Work out the finished part from the listing and answer in its coordinate system (mm). A direction names the side the tool comes from. Coordinates: 2 decimals unless noted, no trailing zeros. Order: outer loops, then holes, each group sorted by start corner. A loop starts at its lowest first (then second) coordinate and runs counter-clockwise, first axis right, second up. Notation, with made-up numbers: (32.5, 59) -> (59.5, 59) arc R29 cw to (59.5, 83) -> close; hole circle Ø6 at (66, -10.5). An arc over 180 degrees is marked (long way). Answer as CSV lines item,"result". Start each with the question number.
Item 1: Section A-A (y = -1.75) is taken. Write down the section's boundary in (x, z) (3 decimals).
Item 2: For a pull along Z with two mould halves and no side action, classify faces 1 (the face through (2.244, -4.072, 8.875)), 2 (the face through (6, -3, -28.575)), 3 (the face through (-5.08, -2, -5)) as pulls with the +Z half, pulls with the -Z half, needs draft (parallel to the pull), parting line crosses it, or undercut.
Item 3: Section D-D (y = 6.5) is taken. Write down the section's boundary in (x, z) (3 decimals).
Item 4: Which of the six approach directions +Z, -Z, +X, -X, +Y, -Y give full straight-line access (tool end or side, diameter ignored) to faces 4 (the face through (-4.765, -3, -23)), 5 (the face through (-4.765, 6, 16)), 6 (the face through (-0.11, -2, -11.43))?
Item 5: Section B-B (z = -7.5) is taken. Write down the section's boundary in (x, y).
Item 6: Straight lines are drawn through the part: L1, parallel to X at y = 2, z = 14.5 (3 decimals); L2, parallel to Y at x = 8.4, z = 0 (3 decimals); L3, parallel to Z at x = -3.25, y = -5.25 (3 decimals). For each, find the intervals that lie inside material, in ascending order.
Item 7: Section C-C (x = 0) is taken. Write down the section's boundary in (y, z) (3 decimals), then the cut area to 3 significant figures.
Item 8: Each of these flat-tipped pins is pushed along its axis until it touches: pin 1 Ø1 at (x, y) = (-2.5, -5.5) entering from -Z (3 decimals); pin 2 Ø6 at (x, y) = (-1.5, 7) entering from +Z (3 decimals); pin 3 Ø1 at (x, z) = (5.5, -19) entering from +Y. Where does it stop, or does it pass through?
```python
from build123d import *
from OCP.BRepFilletAPI import BRepFilletAPI_MakeChamfer

# Parameters (mm, degrees)
SKETCH1_R           = 4.765
BOSS_EXTRUDE1_DEPTH = 9.5
CHAMFER1_SIZE       = 2.54
CHAMFER1_SIZE2      = 7.62
CHAMFER2_SIZE       = 7.62
CHAMFER2_SIZE2      = 2.54
CUT_EXTRUDE1_DEPTH  = 17.5
SKETCH3_W           = 9.53
SKETCH3_H           = 9.53
CUT_EXTRUDE2_DEPTH  = 17.5
SKETCH4_R           = 1.59
CUT_EXTRUDE3_DEPTH  = 17.5


with BuildPart() as part:
    # Sketch1 → Boss-Extrude1 (new, symmetric)
    with BuildSketch(Plane(origin=(0, 0, 0), x_dir=(0, 0, -1), z_dir=(1, 0, 0))):
        with BuildLine():
            Line((0, 9.765), (-22.225, 9.765))
            Line((-22.225, 9.765), (-22.225, 4.765))
            Line((-22.225, 4.765), (-9.705896356, -1.072753903))
            ThreePointArc((-9.705896356, -1.072753903), (-4.321191132, -8.756856297), (5.053224579, -8.355845041))
            Line((5.053224579, -8.355845041), (28.575, -5))
            Line((28.575, -5), (28.575, 0))
            Line((28.575, 0), (9.765, 0))
            ThreePointArc((9.765, 0), (6.904897718, 6.904897718), (0, 9.765))
        make_face()
        Circle(SKETCH1_R, mode=Mode.SUBTRACT)
    extrude(amount=BOSS_EXTRUDE1_DEPTH, both=True)

    # Chamfer1: one chamfer whose edges measure the first distance from different faces: ONE call of the kernel's chamfer builder (chamfer() names one face for all edges)
    chamfer1_edges_1 = [part.edges().sort_by_distance(p)[0] for p in [
        (9.5, 7.265, 22.225),
    ]]
    chamfer1_side_1 = [part.faces().sort_by_distance(p)[0] for p in [
        (0, 7.265, 22.225),
    ]]
    chamfer1_edges_2 = [part.edges().sort_by_distance(p)[0] for p in [
        (9.5, -2.5, -28.575),
    ]]
    chamfer1_side_2 = [part.faces().sort_by_distance(p)[0] for p in [
        (0, -2.5, -28.575),
    ]]
    chamfer1 = BRepFilletAPI_MakeChamfer(part.part.solid().wrapped)
    for e in chamfer1_edges_1:
        chamfer1.Add(CHAMFER1_SIZE, CHAMFER1_SIZE2, e.wrapped, chamfer1_side_1[0].wrapped)  # the first distance lies on this face
    for e in chamfer1_edges_2:
        chamfer1.Add(CHAMFER1_SIZE, CHAMFER1_SIZE2, e.wrapped, chamfer1_side_2[0].wrapped)  # the first distance lies on this face
    add(Compound.cast(chamfer1.Shape()), mode=Mode.REPLACE)

    # Chamfer2
    chamfer2_edges = [part.edges().sort_by_distance(p)[0] for p in [
        (-9.5, 7.265, 22.225),
        (-9.5, -2.5, -28.575),
    ]]
    chamfer2_side = [part.faces().sort_by_distance(p)[0] for p in [
        (-9.5, 9.220751812, 11.1125),
    ]]
    chamfer(chamfer2_edges, length=CHAMFER2_SIZE, length2=CHAMFER2_SIZE2, reference=chamfer2_side[0])

    # Sketch2 → Cut-Extrude1 (cut, symmetric)
    with BuildSketch(Plane(origin=(0, 0, 0), x_dir=(1, 0, 0), z_dir=(0, 1, 0))):
        with BuildLine():
            Line((-5.08, -3.81), (-5.08, 6.35))
            ThreePointArc((-5.08, 6.35), (0, 11.43), (5.08, 6.35))
            Line((5.08, 6.35), (5.08, -3.81))
            ThreePointArc((5.08, -3.81), (0, -8.89), (-5.08, -3.81))
        make_face()
    extrude(amount=CUT_EXTRUDE1_DEPTH, both=True, mode=Mode.SUBTRACT)

    # Sketch3 → Cut-Extrude2 (cut, symmetric)
    with BuildSketch(Plane(origin=(0, 0, 0), x_dir=(1, 0, 0), z_dir=(0, 1, 0))):
        with Locations((0, 23.81)):
            Rectangle(SKETCH3_W, SKETCH3_H)
        with Locations((0, -17.46)):
            Rectangle(SKETCH3_W, SKETCH3_H)
    extrude(amount=CUT_EXTRUDE2_DEPTH, both=True, mode=Mode.SUBTRACT)

    # Sketch4 → Cut-Extrude3 (cut, symmetric)
    with BuildSketch(Plane(origin=(0, 0, 0), x_dir=(0, 0, -1), z_dir=(1, 0, 0))):
        with Locations((26.035, -2.54)):
            Circle(SKETCH4_R)
        with Locations(Location((-19.685, 7.225, 0), (0, 0, 180))):
            Circle(SKETCH4_R)
    extrude(amount=CUT_EXTRUDE3_DEPTH, both=True, mode=Mode.SUBTRACT)


solid = part.part
```
Checked values:
1,outline,"(-9.5, -20.955) -> (-8.267, -24.655) -> (-4.765, -24.655) -> (-4.765, -19.045) -> (4.765, -19.045) -> (4.765, -24.655) -> (8.267, -24.655) -> (9.5, -20.955) -> (9.5, -4.432) -> (5.08, -4.432) -> (5.08, -6.35) arc R5.08 cw to (-5.08, -6.35) -> (-5.08, -4.432) -> (-9.5, -4.432) -> close; (-9.5, 4.432) -> (-5.042, 4.432) arc R5.08 cw to (5.042, 4.432) -> (9.5, 4.432) -> (9.5, 9.607) -> (-9.5, 9.607) -> close; (-7.347, -27.415) -> (-6.96, -28.575) -> (-4.765, -28.575) -> (-4.765, -27.415) -> close; (4.765, -28.575) -> (6.96, -28.575) -> (7.347, -27.415) -> (4.765, -27.415) -> close"
2,face 1,"parting line crosses it"
2,face 2,"pulls with the -Z half"
2,face 3,"undercut"
3,outline,"(-9.5, -7.287) -> (-4.993, -7.287) arc R5.08 cw to (-5.08, -6.35) -> (-5.08, 3.81) arc R5.08 cw to (5.08, 3.81) -> (5.08, -6.35) arc R5.08 cw to (4.993, -7.287) -> (9.5, -7.287) -> (9.5, 14.605) -> (8.278, 18.27) -> (4.765, 18.27) -> (4.765, 12.695) -> (-4.765, 12.695) -> (-4.765, 18.27) -> (-8.278, 18.27) -> (-9.5, 14.605) -> close; (-7.335, 21.1) -> (-4.765, 21.1) -> (-4.765, 22.225) -> (-6.96, 22.225) -> close; (4.765, 21.1) -> (7.335, 21.1) -> (6.96, 22.225) -> (4.765, 22.225) -> close"
4,face 4,"-Z, +Y, -Y"
4,face 5,"+Z, +Y, -Y"
4,face 6,"+Y, -Y"
5,outline,"(-9.5, -8.01) -> (-4.95, -8.01) -> (-4.95, 6.25) -> (-9.5, 6.25) -> close; (4.95, -8.01) -> (9.5, -8.01) -> (9.5, 6.25) -> (4.95, 6.25) -> close"
6,L1,"x = -9.5 to -4.765, 4.765 to 9.5"
6,L2,"y = -9.765 to -4.765, 4.765 to 9.765"
6,L3,"z = -19.045 to -10.254, 7.714 to 8.234"
7,outline,"(-7.446, -11.43) -> (-6.36, -19.045) -> (0, -19.045) -> (0, -11.43) -> close; (-4.04, 8.89) -> (9.765, 8.89) -> (9.765, 12.695) -> (0.321, 12.695) -> (-1.073, 9.706) arc R9.765 ccw to start"
7,area,"93.2 mm^2"
8,pin 1,"stops at z = -19.045"
8,pin 2,"stops at z = 12.695"
8,pin 3,"stops at y = 0"
